Could you check a few things on this model? Use its own coordinates, in mm. A direction names the side the tool comes from. Round coordinates to 2 decimals unless told otherwise and drop trailing zeros. Loops run counter-clockwise (first coordinate to the right, second up) from the corner with the lowest first, then second, coordinate; pieces in that order, holes last. Notation, with made-up numbers: M -28.75,87.5 L 22.25,87.5 A11 cw 22.25,98.5 Z; hole C 21,35 d5. An arc over 180 degrees is marked long. Return JSON: item names as keys, results as strings. Group by question number.
```python
from build123d import *

# Parameters (mm, degrees)
ESQUISSE1_R                  = 9
ESQUISSE1_R_2                = 1.5
BOSS_EXTRU_1_DEPTH           = 20
ESQUISSE2_R                  = 4
ESQUISSE2_R_2                = 3.19
BOSS_EXTRU_2_DEPTH           = 15
CONG_1_R                     = 0.25
CONG_2_R                     = 1
CONG_3_R                     = 1
ENL_V_MAT_EXTRU_1_DEPTH      = 10
ENL_V_MAT_EXTRU_1_DEPTH_BACK = 10
ESQUISSE3_R                  = 1.5
ESQUISSE4_R                  = 1.5
ENL_V_MAT_EXTRU_2_DEPTH      = 10


with BuildPart() as part:
    # Esquisse1 → Boss.-Extru.1 (new body)
    with BuildSketch(Plane.XY):
        Circle(ESQUISSE1_R)
        with Locations((0, 6)):
            Circle(ESQUISSE1_R_2, mode=Mode.SUBTRACT)
        with Locations((6, 0)):
            Circle(ESQUISSE1_R_2, mode=Mode.SUBTRACT)
        with Locations((0, -6)):
            Circle(ESQUISSE1_R_2, mode=Mode.SUBTRACT)
        with Locations((-6, 0)):
            Circle(ESQUISSE1_R_2, mode=Mode.SUBTRACT)
    extrude(amount=BOSS_EXTRU_1_DEPTH)

    # Esquisse2 → Boss.-Extru.2 (add)
    with BuildSketch(Plane(origin=(0, 0, 0), x_dir=(-1, 0, 0), z_dir=(0, 0, -1))):
        with Locations(Location((0, 0, 0), (0, 0, 180))):
            Circle(ESQUISSE2_R)
        Circle(ESQUISSE2_R_2, mode=Mode.SUBTRACT)
    extrude(amount=BOSS_EXTRU_2_DEPTH)

    # Cong_1
    cong_1_edges = [part.edges().sort_by_distance(p)[0] for p in [
        (-4, 0, 0),
    ]]
    fillet(cong_1_edges, radius=CONG_1_R)

    # Cong_2
    cong_2_edges = [part.edges().sort_by_distance(p)[0] for p in [
        (-9, 0, 20),
    ]]
    fillet(cong_2_edges, radius=CONG_2_R)

    # Cong_3
    cong_3_edges = [part.edges().sort_by_distance(p)[0] for p in [
        (-9, 0, 0),
    ]]
    fillet(cong_3_edges, radius=CONG_3_R)

    # Esquisse3 → Enl_v. mat.-Extru.1 (cut, two sides: drawn at the far end of the back side and taken through both)
    with BuildSketch(Plane(origin=(0, 0, 0), x_dir=(1, 0, 0), z_dir=(0, 1, 0)).offset(-ENL_V_MAT_EXTRU_1_DEPTH_BACK)):
        with Locations(Location((0, 7.5, 0), (0, 0, 90))):
            Circle(ESQUISSE3_R)
    extrude(amount=ENL_V_MAT_EXTRU_1_DEPTH + ENL_V_MAT_EXTRU_1_DEPTH_BACK, mode=Mode.SUBTRACT)

    # Esquisse4 → Enl_v. mat.-Extru.2 (cut)
    with BuildSketch(Plane.XY.offset(20)):
        Circle(ESQUISSE4_R)
    extrude(amount=-ENL_V_MAT_EXTRU_2_DEPTH, mode=Mode.SUBTRACT)


solid = part.part
```
1. If we section it at A-A, the plane z = -7.5: Please give me the cut outline in (x, y), then the cut area to 3 significant figures.
2. I need wall thicknesses on probe 1 along Y at (x, z) = (0, 16); probe 2 along Y at (x, z) = (0, 8.5); probe 3 along Z at (x, y) = (-1, 1.5). Which ranges of each line are inside material? Lowest first, please.
3. I'm going to push flat-ended pins straight in: pin 1 Ø10 at (x, z) = (6.5, 12) entering from +Y; pin 2 Ø2.5 at (x, y) = (0, 6) entering from -Z; pin 3 Ø3 at (y, z) = (5, 16) entering from -X; pin 4 Ø4 at (x, z) = (-2.5, 11.5) entering from -Y. Where does each tip first touch, or does it pass through?
4. On a 3-axis mill with a long thin cutter (end or side, diameter ignored), from which of +Z, -Z, +X, -X, +Y, -Y can I reach the whole of each face in a straight line? I mean faces 4 (the face through (-0.325, -7.464, 9.86)), 5 (the face through (0, 0, 10)), 6 (the face through (3.4, -3.4, 0)). Say none if no direction works.
5. We'd pull the mould along X, two halves only. Please class faces 1 (the face through (0, 0, 0)), 2 (the face through (3.695, 1.532, -7.522)), 3 (the face through (0, -2, 20)): +X half, -X half, draft (parallel to the pull), parting line (faces both ways), or undercut.
6. If we section it at B-B, the plane z = 18.5: Please give me the cut outline in (x, y).
7. If we section it at C-C, the plane x = 0: Give the number of separate pieces and of enclosed holes in the cut face, then the cut area to 3 significant figures.
Geometry results:
{
 "1": {"outline": "M -1.5,-3.71 L -1.5,-2.82 A3.19 cw -1.5,2.82 L -1.5,3.71 A4 ccw Z; M 1.5,-3.71 A4 ccw 1.5,3.71 L 1.5,2.82 A3.19 cw 1.5,-2.82 Z", "area": "13.3 mm^2"},
 "2": {"probe 1": "-9 to -7.5, -4.5 to -1.5, 1.5 to 4.5, 7.5 to 9", "probe 2": "-9 to -7.5, -4.5 to 4.5, 7.5 to 9", "probe 3": "0 to 20"},
 "3": {"pin 1": "y = 8.87", "pin 2": "through", "pin 3": "x = -8.29", "pin 4": "y = -8.99"},
 "4": {"face 4": "+Z, -Z", "face 5": "+Z", "face 6": "-Z"},
 "5": {"face 1": "undercut", "face 2": "parting line", "face 3": "draft"},
 "6": {"outline": "C 0,0 d18; hole C -6,0 d3; hole C 0,-6 d3; hole C 0,0 d3; hole C 0,6 d3; hole C 6,0 d3"},
 "7": {"separate pieces": "5", "enclosed holes": "0", "area": "229 mm^2"}
}
